Here's how the part is built. I have some questions about the finished solid (model axes, mm). A direction names the side the tool comes from. Coordinates: 2 decimals unless noted, no trailing zeros. Loops run counter-clockwise (first coordinate to the right, second up) from the corner with the lowest first, then second, coordinate; pieces in that order, holes last. Notation, with made-up numbers: M -25.5,68.25 L -10.5,68.25 A22 cw -10.5,101.25 Z; hole C 17,58 d11. An arc over 180 degrees is marked long. Use one line per item in the form item = value. Start each with the question number.
(1) Imagine slicing it at A-A, the plane x = -19.55. Please give me the cut outline in (y, z).
(2) Will these pins go through, and if not, where does the flat tip stop? P1, Ø2.5, axis at x = -19.55, z = 0, coming from the -Y side; P2, Ø2.5, axis at x = -5.5, y = -25.5, coming from the -Z side; P3, Ø1.1, axis at x = -21, y = -7.5, coming from the +Z side.
(3) Please list where these lines run through material, in increasing order: L1, parallel to X at y = 1.9, z = 0; L2, parallel to Y at x = -10.5, z = -0.25.
(4) Imagine slicing it at B-B, the plane x = 0. Please give me the cut outline in (y, z).
(5) Imagine slicing it at D-D, the plane x = 8.25. Please give me the cut outline in (y, z), and give its area (3 significant figures).
(6) Imagine slicing it at C-C, the plane z = 3.75. Please give me the cut outline in (x, y).
(7) On a 3-axis mill with a long thin cutter (end or side, diameter ignored), from which of +Z, -Z, +X, -X, +Y, -Y can I reach the whole of each face in a straight line? I mean faces 1 (the flat face through (5.75, -10, 0)), 2 (the flat face through (-17.15, -17, 0)), 3 (the flat face through (-17.05, -5.5, -0.1)), 4 (the cylindrical face through (-0.54, 1.97, -2.44)), 5 (the flat face through (-17.05, -10, 0)). Say none if no direction works.
(8) Thinking about a two-plate mould opening in Z: for faces 6 (the flat face through (10.45, -23, 1)), 7 (the cylindrical face through (7.25, -7.38, -0.03)), 8 (the flat face through (-5, -8, -6)), 9 (the cylindrical face through (-8.7, -2.5, -0.1)), which applies, +Z half, -Z half, draft (parallel to the pull), parting line (faces both ways), or undercut?
Autodesk Fusion 360 part; units mm, degrees
sketch "ServoRotatingPlate" plane through (0, 0, 0) normal (0, 1, 0) x (1, 0, 0)
  circle A0 centre (0, 0) radius 5.8
  line L0 (5.75, 6) -> (-17.05, 6)
  line L1 (-17.05, 6) -> (-17.05, -6)
  line L2 (-17.05, -6) -> (5.75, -6)
  line L3 (5.75, -6) -> (5.75, 6)
  line L4 (-8.7, 0) -> (5.75, 0) construction
  circle A1 centre (-6.2, 0) radius 2.5
  circle A2 centre (0, 0) radius 2.5
  circle A3 centre (0, 0) radius 1.1
  point P0 (5.8, 0)
  dimension "d4" = 11.6
  dimension "d6" = 12
  dimension "d7" = 22.8
  dimension "d10" = 5
  dimension "d12" = 14.5
  dimension "d13" = 5.75
  dimension "d14" = 8.1
  dimension "d48" = 5
  dimension "d49" = 1.4
extrude "Extrude1" add sketch "ServoRotatingPlate" against normal blind 5 contours A0 L3 | A0 L3 A1 | A0 A1 | A0 A1 | A2 | A3
extrude "Extrude2" add sketch "ServoRotatingPlate" against normal blind 22.5 from surface at -5 contours A0 L3 A1 | A0 L0 L1 L2 L3 A1 | A0 A1 | A0 A1 | A2 | A3
ref_plane "WorkPlane1" through (-5.65, -6, 0) normal (0, 1, 0) x (0, 0, 1)
sketch "EarBase" plane through (-5.65, -6, 0) normal (0, 1, 0) x (1, 0, 0)
  line L0 (16.1, 6) -> (-16.1, 6)
  line L1 (-16.1, 6) -> (-16.1, -6)
  line L2 (-16.1, -6) -> (16.1, -6)
  line L3 (16.1, -6) -> (16.1, 6)
  line L4 (16.1, 6) -> (-16.1, -6) construction
  line L5 (-16.1, 6) -> (16.1, -6) construction
  line L6 (-16.1, 0) -> (16.1, 0) construction
  circle A0 centre (-13.9, 0) radius 1
  line L7 (-14.7, 0.6) -> (-16.1, 0.6)
  line L8 (-14.7, -0.6) -> (-16.1, -0.6)
  line L9 (-11.4, 6) -> (-11.4, -6)
  line L10 (0, 0) -> (0, 6) construction
  line L11 (14.7, 0.6) -> (16.1, 0.6)
  circle A1 centre (13.9, 0) radius 1
  line L12 (14.7, -0.6) -> (16.1, -0.6)
  point P0 (11.4, 6)
  dimension "d26" = 32.2
  dimension "d31" = 2
  dimension "d33" = 1.2
  dimension "d34" = 2.5
  dimension "d35" = 4.7
extrude "Extrude3" add sketch "EarBase" against normal blind 2.8 contours L0 L2 L3 L9 L11 A1 L12 | L0 L1 L2 A0 L7 L8 L9
ref_plane "WorkPlane2" through (-5.65, -22.5, 0) normal (0, -1, 0) x (0, 0, -1)
sketch "StickerBase" plane through (-5.65, -22.5, 0) normal (0, -1, 0) x (1, 0, 0)
  line L0 (11.5, -6.25) -> (-11.5, -6.25)
  line L1 (-11.5, -6.25) -> (-11.5, 6.25)
  line L2 (-11.5, 6.25) -> (11.5, 6.25)
  line L3 (11.5, 6.25) -> (11.5, -6.25)
  line L4 (11.5, -6.25) -> (-11.5, 6.25) construction
  line L5 (-11.5, -6.25) -> (11.5, 6.25) construction
  dimension "d42" = 23
  dimension "d43" = 12.5
extrude "Extrude4" add sketch "StickerBase" against normal blind 10.5
extrude "Extrude5" add sketch "ServoRotatingPlate" along normal blind 4 contours A2
sketch "WireHardCoded" plane through (5.75, 0, 0) normal (1, 0, 0) x (0, 0, -1)
  line L0 (6, -22.5) -> (-6, -22.5)
  line L1 (-6, -22.5) -> (-6, -27.5)
  line L2 (-6, -27.5) -> (6, -27.5)
  line L3 (6, -27.5) -> (6, -22.5)
  line L4 (-1.75, -23.5) -> (1.75, -23.5) construction
  line L5 (1.75, -23.5) -> (1.75, -22.3333) construction
  line L6 (1.75, -22.3333) -> (-1.75, -22.3333) construction
  line L7 (-1.75, -22.3333) -> (-1.75, -23.5) construction
  line L8 (0, -27.5) -> (0, -23.5) construction
  line L9 (-1.75, -22.9167) -> (1.75, -22.9167) construction
  circle A0 centre (0, -22.9167) radius 0.5833
  circle A1 centre (-1.17, -22.9167) radius 0.5833
  circle A2 centre (1.17, -22.9167) radius 0.5833
  dimension "d52" = 1.1667
  dimension "d53" = 3.5
  dimension "d54" = 4
  dimension "d57" = 1.17
  dimension "d58" = 0
extrude "Extrude6" add sketch "WireHardCoded" along normal up to surface (4.7 mm away) contours L0 A2 | L0 A2 | L0 A0 | L0 A0 | L0 A1 | L0 A1
equation "BaseCircleD = 11.6 mm"
equation "d4 = BaseCircleD"
equation "BaseRectW = 12 mm"
equation "d6 = BaseRectW"
equation "d7 = BaseRectH"
equation "BaseRectH = 22.8 mm"
equation "BaseCircle2D = 5 mm"
equation "d10 = BaseCircle2D"
equation "E2EDist = 14.5 mm"
equation "d12 = E2EDist"
equation "d13 = CenterMeasureL"
equation "CenterMeasureL = 5.75 mm"
equation "GearIsleHeight = 5 mm"
equation "BoxHeight = 22.5 mm"
equation "Ear_Down = 1 mm"
equation "Ear_L = 32.2 mm"
equation "d26 = Ear_L"
equation "Ear_Thick = 2.8 mm"
equation "EarScrew_D = 2 mm"
equation "d31 = EarScrew_D"
equation "Ear_Slit = 1.2 mm"
equation "d33 = Ear_Slit"
equation "d34 = HolePos"
equation "HolePos = 2.5 mm"
equation "sticker_height = 10.5 mm"
equation "stick_pos = 5 mm"
equation "Sticker_Profile_L = 23 mm"
equation "Sticker_Profile_W = 12.5 mm"
equation "d42 = Sticker_Profile_L"
equation "d43 = Sticker_Profile_W"
equation "ServoShaftProf = 5 mm"
equation "ServoProfHeight = 4 mm"
equation "d48 = ServoShaftProf"
equation "d50 = ServoProfHeight"
equation "d52 = ( 3.5 / 3 ) * 1 mm"
Answer:
q1.outline = M -8.8,-6 L -6,-6 L -6,-1 L -8.8,-1 Z; M -8.8,1 L -6,1 L -6,6 L -8.8,6 Z
q2.P1 = -8.8
q2.P2 = -6
q2.P3 = 6
q3.L1 = -2.5 to -1.1, 1.1 to 2.5
q3.L2 = -27.5 to -5
q4.outline = M -27.5,-6 L -22.5,-6 L -22.5,-6.25 L -12,-6.25 L -12,-6 L -5,-6 L -5,-5.8 L 0,-5.8 L 0,-2.5 L 4,-2.5 L 4,-1.1 L 0,-1.1 L 0,1.1 L 4,1.1 L 4,2.5 L 0,2.5 L 0,5.8 L -5,5.8 L -5,6 L -12,6 L -12,6.25 L -22.5,6.25 L -22.5,6 L -27.5,6 Z
q5.outline = C -22.92,-1.17 d1.17; C -22.92,0 d1.17; C -22.92,1.17 d1.17; M -8.8,-6 L -6,-6 L -6,-1 L -8.8,-1 Z; M -8.8,1 L -6,1 L -6,6 L -8.8,6 Z
q5.area = 31.2 mm²
q6.outline = M -21.75,-8.8 L -17.05,-8.8 L -17.05,-12 L -17.15,-12 L -17.15,-22.5 L -17.05,-22.5 L -17.05,-27.5 L 5.75,-27.5 L 5.75,-22.5 L 5.85,-22.5 L 5.85,-12 L 5.75,-12 L 5.75,-8.8 L 10.45,-8.8 L 10.45,-6 L 5.75,-6 L 5.75,-5 L 4.42,-5 L 4.42,0 L -4.42,0 L -4.42,-5 L -17.05,-5 L -17.05,-6 L -21.75,-6 Z
q7.face_1 = +Z, -Z, +X
q7.face_2 = +Z, -Z, -X, -Y
q7.face_3 = +Z, -Z, -X, +Y
q7.face_4 = +Y
q7.face_5 = +Z, -Z, -X
q8.face_6 = draft
q8.face_7 = undercut
q8.face_8 = -Z half
q8.face_9 = parting line
